Check sheet for the modelled part. Datum: model origin and axes. Units: mm. Face numbers are marked on the shaded views. A direction names the side the tool comes from. Round coordinates to 2 decimals unless told otherwise and drop trailing zeros. Loops run counter-clockwise (first coordinate to the right, second up) from the corner with the lowest first, then second, coordinate; pieces in that order, holes last. Notation, with made-up numbers: (14.5, -6.75) - (70.5, -6.75) arc R22 ccw to (70.5, 14.25) - close; hole circle Ø11 at (-19.5, 52). An arc over 180 degrees is marked (long way). Answer in a Markdown table with one row per item. Add a question column.
(1) Cross-section at D-D on z = 24. Enter the section's corners in (x, y).
(2) Cross-section at B-B on y = -10. Enter the section's corners in (x, z).
(3) Thickness scan on line 1 along X through (y, z) = (2.5, 10.5); line 2 along Y through (x, z) = (-10, 7.5). Record the ranges inside material, lowest first.
(4) Cross-section at A-A on z = 11.5. Enter the section's corners in (x, y).
(5) Gauge pin test, flat ends, axial feed: pin 1 (1.5 mm diameter, centred on y = -1, z = 12, fed in from -X); pin 2 (2 mm diameter, centred on x = -5.5, z = 30, fed in from -Y); pin 3 (1.5 mm diameter, centred on x = 2, y = 3, fed in from -Z). Record the tip position at first contact, or that the pin passes through.
(6) Cross-section at C-C on x = 2.5. Enter the section's corners in (y, z), then the cut area to 3 significant figures.
(7) Access from +Z, -Z, +X, -X, +Y, -Y to the whole of each face (thin tool, end or side, straight path). Record for the marked faces 1 and 2.
(8) Mould release check, pull along Y, two halves, no side actions. Record for the marked faces 3, 4 and 5: +Y half, -Y half, draft (parallel to the pull), parting line (faces both ways), or undercut.
from build123d import *

# Parameters (mm, degrees)
PAD_DEPTH    = 42
SKETCH001_R  = 1.5
PAD001_DEPTH = 3
SKETCH002_R  = 1.5
POCKET_DEPTH = 15


with BuildPart() as part:
    # Sketch → Pad (new body)
    with BuildSketch(Plane.XY):
        Polygon((0, 0), (0, -15), (5, -15), (5, 5), (-15, 5), (-15, 0), align=None)
    extrude(amount=PAD_DEPTH)

    # Sketch001 (on Face8 of Pad) → Pad001 (join)
    with BuildSketch(Plane.XY.offset(42)):
        with Locations((-10, 2.5)):
            Circle(SKETCH001_R)
        with Locations((2.5, 2.5)):
            Circle(SKETCH001_R)
        with Locations((2.5, -10)):
            Circle(SKETCH001_R)
    extrude(amount=PAD001_DEPTH)

    # Sketch002 (on Face4 of Pad001) → Pocket (cut)
    with BuildSketch(Plane(origin=(0, 0, 0), x_dir=(1, 0, 0), z_dir=(0, 0, -1))):
        with Locations((2.5, -2.5)):
            Circle(SKETCH002_R)
        with Locations((2.5, 10)):
            Circle(SKETCH002_R)
        with Locations((-10, -2.5)):
            Circle(SKETCH002_R)
    extrude(amount=-POCKET_DEPTH, mode=Mode.SUBTRACT)


solid = part.part
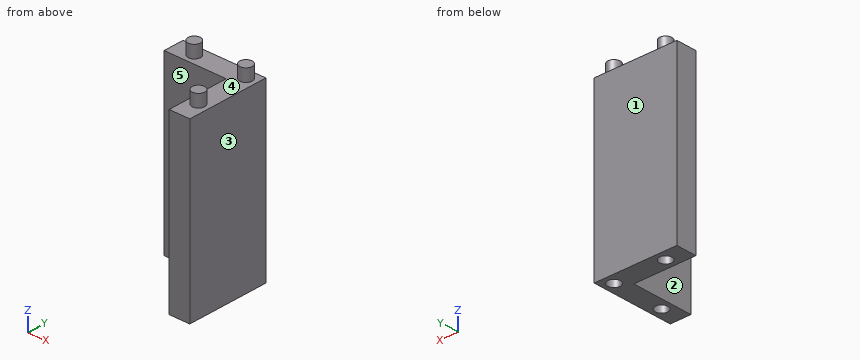
Answers:
| question | item | result |
|---|---|---|
| 1 | outline | (-15, 0) - (0, 0) - (0, -15) - (5, -15) - (5, 5) - (-15, 5) - close |
| 2 | outline | (0, 0) - (1, 0) - (1, 15) - (4, 15) - (4, 0) - (5, 0) - (5, 42) - (4, 42) - (4, 45) - (1, 45) - (1, 42) - (0, 42) - close |
| 3 | line 1 | x = -15 to -11.5, -8.5 to 1, 4 to 5 |
| 3 | line 2 | y = 0 to 1, 4 to 5 |
| 4 | outline | (-15, 0) - (0, 0) - (0, -15) - (5, -15) - (5, 5) - (-15, 5) - close; hole circle Ø3 at (-10, 2.5); hole circle Ø3 at (2.5, -10); hole circle Ø3 at (2.5, 2.5) |
| 5 | pin 1 | stops at x = 0 |
| 5 | pin 2 | stops at y = 0 |
| 5 | pin 3 | stops at z = 15 |
| 6 | outline | (-15, 0) - (-11.5, 0) - (-11.5, 15) - (-8.5, 15) - (-8.5, 0) - (1, 0) - (1, 15) - (4, 15) - (4, 0) - (5, 0) - (5, 42) - (4, 42) - (4, 45) - (1, 45) - (1, 42) - (-8.5, 42) - (-8.5, 45) - (-11.5, 45) - (-11.5, 42) - (-15, 42) - close |
| 6 | area | 768 mm^2 |
| 7 | face 1 | +Z, -Z, +X, -X, +Y |
| 7 | face 2 | +Z, -Z, -X, -Y |
| 8 | face 3 | draft |
| 8 | face 4 | undercut |
| 8 | face 5 | -Y half |
